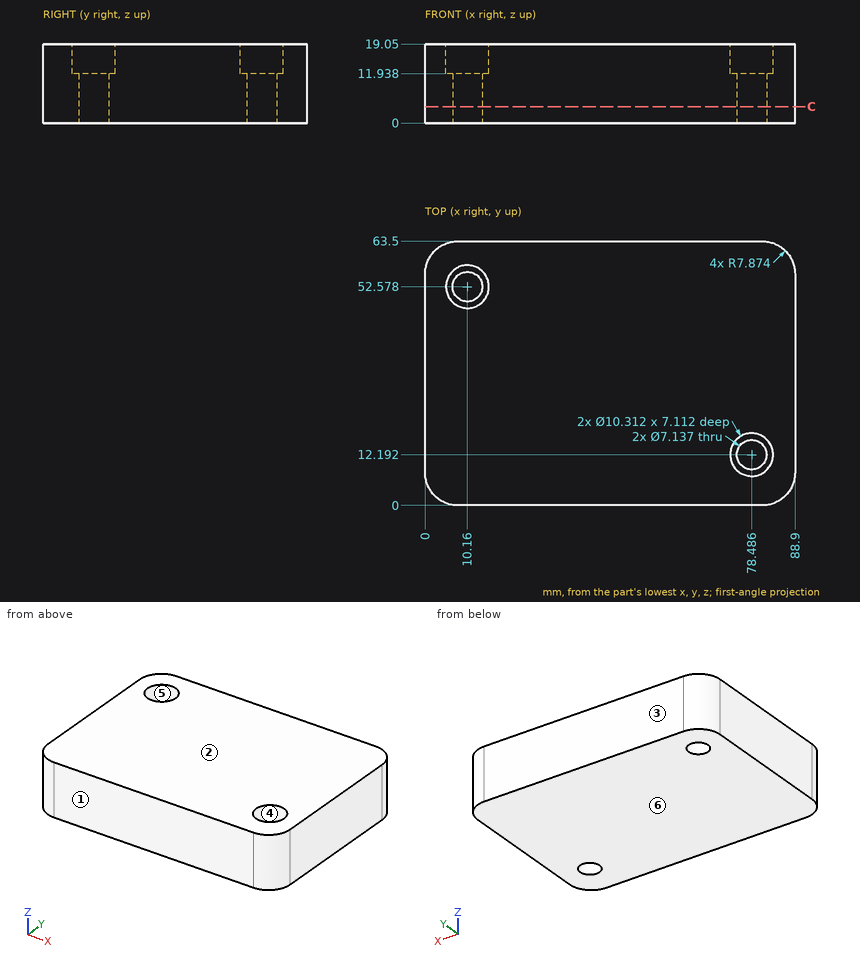
Study the drawing (mm; zero at the part's minimum x, y, z) and answer. A direction names the side the tool comes from. Give positions to 0.01 mm unless a question says otherwise; leave off trailing zeros. Order: outer loops, then holes, each group sorted by start corner. A loop starts at its lowest first (then second) coordinate and runs counter-clockwise, first axis right, second up. Notation, with made-up numbers: (-22, 16) - (19, 16) arc R18 ccw to (19, 27) - close; hole circle Ø9 at (65.25, -1). An arc over 180 degrees is marked (long way). Answer in a Markdown table with one row per item. Add a question column.
Q1. The part is cut by section C-C (z = 4). Determine the outline of the cut face in (x, y), then the cut area to 3 significant figures.
Q2. Given P1, Ø5.5, axis at x = 10.16, y = 52.578, coming from the +Z side, flat-ended and moving along its own axis, determine where the tip first touches the part or whether it passes through.
Q3. Find the intervals of material crossed by line 1 along Y through (x, z) = (10.16, 17.5) (1 decimal); line 2 along X through (y, z) = (10.5, 13.75) (1 decimal); line 3 along X through (y, z) = (13, 4.5), in increasing order. Write a range as [from, to].
Q4. For a pull along Y with two mould halves and no side action, classify the marked faces 1, 2, 3 and 4 as released by +Y, released by -Y, zero draft, split by the parting line, or undercut.
Q5. Which of the six approach directions +Z, -Z, +X, -X, +Y, -Y give full straight-line access (tool end or side, diameter ignored) to the marked faces 5 and 6?
Determined:
| question | item | result |
|---|---|---|
| 1 | outline | (0, 7.87) arc R7.87 ccw to (7.87, 0) - (81.03, 0) arc R7.87 ccw to (88.9, 7.87) - (88.9, 55.63) arc R7.87 ccw to (81.03, 63.5) - (7.87, 63.5) arc R7.87 ccw to (0, 55.63) - close; hole circle Ø7.14 at (10.16, 52.58); hole circle Ø7.14 at (78.49, 12.19) |
| 1 | area | 5,510 mm² |
| 2 | P1 | passes through |
| 3 | line 1 | y = [0, 47.4], [57.7, 63.5] |
| 3 | line 2 | x = [0, 73.6], [83.4, 88.9] |
| 3 | line 3 | x = [0, 75.01], [81.96, 88.9] |
| 4 | face 1 | released by -Y |
| 4 | face 2 | zero draft |
| 4 | face 3 | released by +Y |
| 4 | face 4 | undercut |
| 5 | face 5 | +Z |
| 5 | face 6 | -Z, +X, -X, +Y, -Y |
